```python
from build123d import *

# Parameters (mm, degrees)
HOLE1_D                      = 6
HOLE1_DEPTH                  = 15.2664
HOLE1_CBORE_D                = 10
HOLE1_CBORE_DEPTH            = 4
CHAMFER1_SIZE                = 0.635
CIRPATTERN1_COUNT            = 10
CHAMFER1_OF_CIRPATTERN1_SIZE = 0.635
FILLET1_R                    = 1.27


with BuildPart() as part:
    # Sketch1 → Revolve1 (revolve)
    with BuildSketch(Plane.XY):
        Polygon((8.89, 0), (45.085, 0), (45.085, -15.2654), (24.13, -15.2654), (24.13, -6.35), (8.89, -6.35), align=None)
    revolve(axis=Axis((0, 0, 0), (0, 1, 0)))

    # Hole1
    with Locations(Plane(origin=(0, 0, 0), x_dir=(1, 0, 0), z_dir=(0, 1, 0))):
        with Locations((38.1, 0)):
            hole1 = CounterBoreHole(HOLE1_D / 2, HOLE1_CBORE_D / 2, HOLE1_CBORE_DEPTH, depth=HOLE1_DEPTH)

    # Chamfer1
    chamfer1_edges = [part.edges().sort_by_distance(p)[0] for p in [
        (33.1, 0, 0),
    ]]
    chamfer(chamfer1_edges, length=CHAMFER1_SIZE)

    # CirPattern1: Hole1 ×10 about axis
    cirpattern1_axis = Axis((0, 0, 0), (0, 1, 0))
    for i in range(1, CIRPATTERN1_COUNT):
        add(hole1.rotate(cirpattern1_axis, i * 360 / CIRPATTERN1_COUNT), mode=Mode.SUBTRACT)

    # Chamfer1 of CirPattern1
    chamfer1_of_cirpattern1_edges = [part.edges().sort_by_distance(p)[0] for p in [
        (26.778462514, 0, -19.455691851),
        (10.228462514, 0, -31.479970689),
        (-10.228462514, 0, -31.479970689),
        (-26.778462514, 0, -19.455691851),
        (-33.1, 0, 0),
        (-26.778462514, 0, 19.455691851),
        (-10.228462514, 0, 31.479970689),
        (10.228462514, 0, 31.479970689),
        (26.778462514, 0, 19.455691851),
    ]]
    chamfer(chamfer1_of_cirpattern1_edges, length=CHAMFER1_OF_CIRPATTERN1_SIZE)

    # Fillet1
    fillet1_edges = [part.edges().sort_by_distance(p)[0] for p in [
        (-24.13, -6.35, 0),
    ]]
    fillet(fillet1_edges, radius=FILLET1_R)


solid = part.part
```
Geometry: final body of the model. Coordinates: model frame, mm. A direction names the side the tool comes from. Give positions to 0.01 mm unless a question says otherwise; leave off trailing zeros. Order: outer loops, then holes, each group sorted by start corner. A loop starts at its lowest first (then second) coordinate and runs counter-clockwise, first axis right, second up. Notation, with made-up numbers: (-19, 14.5) -> (2, 14.5) arc R25 ccw to (2, 49.5) -> close; hole circle Ø3 at (-8, -28.5). An arc over 180 degrees is marked (long way). Write each question's results on one line, items separated by ' | '. Start each with the question number.
1) Line query: line 1 (X direction, y = -2, z = 19); line 2 (Z direction, x = 14, y = -8.5); line 3 (X direction, y = -8.75, z = -35). Output: solid intervals per line, ascending. Write a range as from..to.
2) Section B-B (z = 0). Count the separate pieces of the cut face and the enclosed holes in it, then the cut area to 3 significant figures.
3) First-contact query: pin 1 (1.5 mm diameter, centred on y = -7, z = 22, fed in from +X); pin 2 (4 mm diameter, centred on y = -1.5, z = 7.5, fed in from -X); pin 3 (3.5 mm diameter, centred on x = 38.1, z = 0, fed in from -Y); pin 4 (8 mm diameter, centred on x = -11.77, z = 36.24, fed in from +Y). Flat tips, straight axial feed; report the tip coordinate or a pass-through.
4) Section D-D (x = 38.1). Return loops of the section in (y, z) (3 decimals).
5) Draft query along Z for faces 3 (the flat face through (0, -6.35, 10)), 4 (the cylindrical face through (-11.38, -2.29, -41.22)). Return one class per face: pulls with the +Z half, pulls with the -Z half, needs draft (parallel to the pull), parting line crosses it, or undercut.
6) Set-up query: faces 1 (the cylindrical face through (35.24, -9.71, -0.9)), 2 (the flat face through (15, -4, -35)). Return all of +Z, -Z, +X, -X, +Y, -Y with unobstructed straight access to the full face (end or side cutting, diameter ignored); none if empty.
7) Section A-A (x = 0). Return loops of the section in (y, z) (3 decimals), then the cut area to 3 significant figures.
Calculated:
1) line 1: -40.89..-34.49, -27.15..27.15, 34.49..40.89 | line 2: -42.86..-38.25, -34.22..-19.65, 19.65..34.22, 38.25..42.86 | line 3: -28.42..-14.51, -9.04..9.04, 14.51..28.42
2) separate pieces: 4 | enclosed holes: 0 | area: 618 mm2
3) pin 1: x = 39.76 | pin 2: x = -44.75 | pin 3: through | pin 4: y = -4
4) outline: (-15.265, -24.105) -> (0, -24.105) -> (0, -5.635) -> (-0.635, -5) -> (-4, -5) -> (-4, -3) -> (-15.265, -3) -> close; (-15.265, 3) -> (-4, 3) -> (-4, 5) -> (-0.635, 5) -> (0, 5.635) -> (0, 24.105) -> (-15.265, 24.105) -> close
5) face 3: undercut | face 4: undercut
6) face 1: +Y, -Y | face 2: +Y
7) outline: (-15.265, -45.085) -> (0, -45.085) -> (0, -8.89) -> (-6.35, -8.89) -> (-6.35, -22.86) arc R1.27 cw to (-7.62, -24.13) -> (-15.265, -24.13) -> close; (-15.265, 24.13) -> (-7.62, 24.13) arc R1.27 cw to (-6.35, 22.86) -> (-6.35, 8.89) -> (0, 8.89) -> (0, 45.085) -> (-15.265, 45.085) -> close | area: 834 mm2
